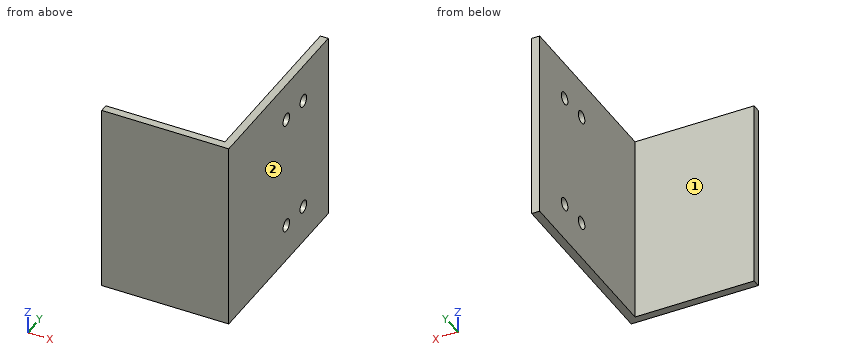
Autodesk Inventor part; units mm, degrees
ref_plane "YZ Plane" through (0, 0, 0) normal (1, 0, 0) x (0, 1, 0)
ref_plane "XZ Plane" through (0, 0, 0) normal (0, 1, 0) x (-1, 0, 0)
ref_plane "XY Plane" through (0, 0, 0) normal (0, 0, 1) x (1, 0, 0)
sketch "Sketch1" plane through (0, 0, 0) normal (0, 1, 0) x (-1, 0, 0)
  line L0 (0, 0) -> (50.8, 0)
  line L1 (50.8, 0) -> (50.8, -76.2)
  line L2 (50.8, -76.2) -> (0, -76.2)
  line L3 (0, -76.2) -> (0, 0)
  dimension "d0" = 50.8
  dimension "d1" = 76.2
extrude "Extrusion1" add sketch "Sketch1" along normal blind 76.2
shell "Shell1" thickness 3.175 removed faces 4 at (-33.8667, 25.4, 0) at (-50.8, 25.4, -50.8) at (-16.9333, 25.4, -76.2) at (-33.8667, 76.2, -50.8)
sketch "Sketch2" plane through (-3.175, 3.175, 0) normal (-1, 0, 0) x (0, 0, 1)
  circle A0 centre (-15.1, 40.925) radius 2.5
  circle A1 centre (-61.1, 53.925) radius 2.5
  circle A2 centre (-61.1, 40.925) radius 2.5
  circle A3 centre (-15.1, 53.925) radius 2.5
  line L0 (-61.1, 53.925) -> (-15.1, 53.925) construction
  line L1 (-15.1, 53.925) -> (-15.1, 40.925) construction
  line L2 (-15.1, 40.925) -> (-61.1, 40.925) construction
  line L3 (-61.1, 40.925) -> (-61.1, 53.925) construction
  line L4 (0, 0) -> (-76.2, 0)
  point P0 (0, -3.175)
  point P1 (-38.1, 53.925)
  point P2 (-38.1, 0)
  dimension "d5" = 5
  dimension "d6" = 46
  dimension "d7" = 13
  dimension "d8" = 40.925
extrude "Extrusion2" cut sketch "Sketch2" against normal blind 25.4
properties part number "BK10_Z_Mount"
The model under review builds one solid part; all positions refer to its coordinate system, in mm. Face numbers are marked on the shaded views. A direction names the side the tool comes from. Round coordinates to 2 decimals unless told otherwise and drop trailing zeros. Loops run counter-clockwise (first coordinate to the right, second up) from the corner with the lowest first, then second, coordinate; pieces in that order, holes last. Notation, with made-up numbers: M -40,29.5 L 7,29.5 A14 ccw 7,50.5 Z; hole C 42,10 d4. An arc over 180 degrees is marked long. Put each result on its own line as item: value.
Q1. Consider section A-A, the plane z = -15.1. Give the boundary of the cut face in (x, y) (3 decimals), then the cut area to 3 significant figures.
Result set:
outline: M -50.8,0 L 0,0 L 0,41.6 L -3.175,41.6 L -3.175,3.175 L -50.8,3.175 Z; M -3.175,46.6 L 0,46.6 L 0,54.6 L -3.175,54.6 Z; M -3.175,59.6 L 0,59.6 L 0,76.2 L -3.175,76.2 Z
area: 361 mm²
Q2. To check wall thickness, follow L1, parallel to Z at x = -1, y = 44; L2, parallel to Y at x = -1.95, z = -61.1; L3, parallel to X at y = 32, z = -58 (3 decimals). State the ranges of each line that lie inside material, in increasing order.
Result set:
L1: z = -76.2 to -63.6, -58.6 to -17.6, -12.6 to 0
L2: y = 0 to 41.6, 46.6 to 54.6, 59.6 to 76.2
L3: x = -3.175 to 0
Q3. For pin 1 (4 mm diameter, centred on x = -22.5, z = -29.5, fed in from -Y); pin 2 (8 mm diameter, centred on x = -8.5, z = -36, fed in from +Y) (3 decimals); pin 3 (6 mm diameter, centred on y = 30.5, z = -44.5, fed in from -X) (3 decimals), all flat-tipped, find the tip position at first contact; note any pin that passes through.
Result set:
pin 1: stops at y = 0
pin 2: stops at y = 3.175
pin 3: stops at x = -3.175
Q4. Machinability: for the marked faces 1 and 2, which of the approach directions +Z, -Z, +X, -X, +Y, -Y give a long, thin tool a straight path to every point of the face, cutting with its end or side? Answer none if there is none.
Result set:
face 1: +Z, -Z, -X, +Y
face 2: +Z, -Z, +X, +Y, -Y
Q5. Consider section C-C, the plane x = -27. Give the boundary of the cut face in (y, z) (3 decimals), then the cut area to 3 significant figures.
Result set:
outline: M 0,-76.2 L 3.175,-76.2 L 3.175,0 L 0,0 Z
area: 242 mm²
Q6. Consider section B-B, the plane y = 57.1. Give the boundary of the cut face in (x, z) (3 decimals).
Result set:
outline: M -3.175,-76.2 L 0,-76.2 L 0,-63.6 L -3.175,-63.6 Z; M -3.175,-58.6 L 0,-58.6 L 0,-17.6 L -3.175,-17.6 Z; M -3.175,-12.6 L 0,-12.6 L 0,0 L -3.175,0 Z
Q7. Consider section D-D, the plane y = 66. Give the boundary of the cut face in (x, z) (3 decimals), then the cut area to 3 significant figures.
Result set:
outline: M -3.175,-76.2 L 0,-76.2 L 0,0 L -3.175,0 Z
area: 242 mm²
